```python
from build123d import *

# Parameters (mm, degrees)
SKETCH2_W                       = 223
SKETCH2_H                       = 222.25
BOSS_EXTRUDE1_DEPTH             = 12.7
FILLET6_R                       = 20
FILLET5_R                       = 3
CBORE_FOR_M3_SBHCS1_D           = 3.4
CBORE_FOR_M3_SBHCS1_DEPTH       = 12.7
CBORE_FOR_M3_SBHCS1_CBORE_D     = 6.7
CBORE_FOR_M3_SBHCS1_CBORE_DEPTH = 3
CBORE_FOR_M5_SBHCS1_D           = 5.5
CBORE_FOR_M5_SBHCS1_DEPTH       = 12.7
CBORE_FOR_M5_SBHCS1_CBORE_D     = 10.5
CBORE_FOR_M5_SBHCS1_CBORE_DEPTH = 5
SKETCH9_R                       = 6.5
CUT_EXTRUDE1_DEPTH              = 2


with BuildPart() as part:
    # Sketch2 → Boss-Extrude1 (new body)
    with BuildSketch(Plane(origin=(0, 0, 0), x_dir=(1, 0, 0), z_dir=(0, 1, 0))):
        Rectangle(SKETCH2_W, SKETCH2_H)
    extrude(amount=BOSS_EXTRUDE1_DEPTH)

    # Fillet6
    fillet6_edges = [part.edges().sort_by_distance(p)[0] for p in [
        (111.5, 6.35, 111.125),
        (111.5, 6.35, -111.125),
    ]]
    fillet(fillet6_edges, radius=FILLET6_R)

    # Fillet5
    fillet5_edges = [part.edges().sort_by_distance(p)[0] for p in [
        (-111.5, 12.7, 0),
        (-10, 12.7, -111.125),
        (-10, 12.7, 111.125),
        (111.5, 12.7, 0),
        (105.642135624, 12.7, 105.267135624),
        (105.642135624, 12.7, -105.267135624),
    ]]
    fillet(fillet5_edges, radius=FILLET5_R)

    # CBORE for M3 SBHCS1
    with Locations(Plane(origin=(0, 12.7, 0), x_dir=(1, 0, 0), z_dir=(0, 1, 0))):
        with Locations((36.5, -98.425), (36.5, 98.425), (19.5, -98.425), (19.5, 98.425), (2.5, -98.425), (2.5, 98.425)):
            CounterBoreHole(CBORE_FOR_M3_SBHCS1_D / 2, CBORE_FOR_M3_SBHCS1_CBORE_D / 2, CBORE_FOR_M3_SBHCS1_CBORE_DEPTH, depth=CBORE_FOR_M3_SBHCS1_DEPTH)

    # CBORE for M5 SBHCS1
    with Locations(Plane(origin=(0, 12.7, 0), x_dir=(1, 0, 0), z_dir=(0, 1, 0))):
        with Locations((-91.5, 98.425), (-91.5, -98.425)):
            CounterBoreHole(CBORE_FOR_M5_SBHCS1_D / 2, CBORE_FOR_M5_SBHCS1_CBORE_D / 2, CBORE_FOR_M5_SBHCS1_CBORE_DEPTH, depth=CBORE_FOR_M5_SBHCS1_DEPTH)

    # Sketch9 → Cut-Extrude1 (cut)
    with BuildSketch(Plane.XZ):
        with Locations((-91.5, 98.425)):
            Circle(SKETCH9_R)
        with Locations((-91.5, -98.425)):
            Circle(SKETCH9_R)
    extrude(amount=-CUT_EXTRUDE1_DEPTH, mode=Mode.SUBTRACT)


solid = part.part
```
Geometry check sheet. Reference: the model listing, model coordinates, mm. A direction names the side the tool comes from. Coordinates: 2 decimals unless noted, no trailing zeros. Answer as a JSON object with one key per item and string values.
1. Draft check along Z on faces 1 (the cylindrical face through (-85.3, 0.99, 100.38)), 2 (the flat face through (-11, 5, -111.125)), 3 (the flat face through (111.5, 5, 1)). Enter one of: released by +Z, released by -Z, zero draft, split by the parting line, or undercut.
Answers below:
{"face 1": "undercut", "face 2": "released by -Z", "face 3": "zero draft"}
2. Section check A-A, the plane x = -91.5. Give the number of separate pieces and of enclosed holes in the cut face, plus the area to 3 significant figures.
Answers below:
{"separate pieces": "3", "enclosed holes": "0", "area": "2,600 mm²"}
3. Go/stop test with flat-tipped pins: pin 1 Ø8.5 at (x, z) = (-91.5, 98.425) entering from -Y; pin 2 Ø5.5 at (x, z) = (36.5, 98.425) entering from +Y; pin 3 Ø9 at (x, z) = (-91.5, -98.425) entering from +Y. Record where each tip stops, or that it passes through.
Answers below:
{"pin 1": "stops at y = 2", "pin 2": "stops at y = 9.7", "pin 3": "stops at y = 7.7"}
4. Tool access check on faces 4 (the cylindrical face through (-89.32, 4.81, -96.75)), 5 (the flat face through (-89, 2, -100)), 6 (the cylindrical face through (39.6, 11.2, 99.7)). Record the directions out of +Z, -Z, +X, -X, +Y, -Y that give a thin tool (end or side, any length) a straight path to the whole face; none if there is none.
Answers below:
{"face 4": "+Y, -Y", "face 5": "-Y", "face 6": "+Y"}
5. Scan lines: L1, parallel to Z at x = 19.5, y = 7.25 (3 decimals); L2, parallel to Z at x = -91.5, y = 9.75 (3 decimals); L3, parallel to X at y = 8, z = 99.5. Record each from-to range of solid material in increasing order.
Answers below:
{"L1": "z = -111.125 to -100.125, -96.725 to 96.725, 100.125 to 111.125", "L2": "z = -111.125 to -103.675, -93.175 to 93.175, 103.675 to 111.125", "L3": "x = -111.5 to -96.64, -86.36 to 1.18, 3.82 to 18.18, 20.82 to 35.18, 37.82 to 109.66"}
